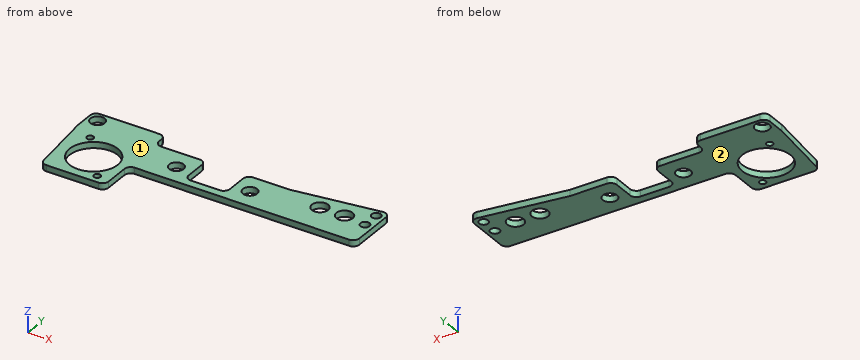
```python
from build123d import *

# Parameters (mm, degrees)
ESQUISSE1_W              = 146
ESQUISSE1_H              = 20
BOSS_EXTRU_1_DEPTH       = 3
ESQUISSE2_R              = 3.5
ENL_V_MAT_EXTRU_3_DEPTH  = 4
ESQUISSE6_W              = 35
ESQUISSE6_H              = 3
BOSS_EXTRU_3_DEPTH       = 8
ESQUISSE8_R              = 3.5
ENL_V_MAT_EXTRU_4_DEPTH  = 8
ESQUISSE7_W              = 35
ESQUISSE7_H              = 3
BOSS_EXTRU_4_DEPTH       = 24
CONG_2_R                 = 3
ESQUISSE10_W             = 20.127249292
ESQUISSE10_H             = 16
ENL_V_MAT_EXTRU_5_DEPTH  = 24
CONG_3_R                 = 3
BOSS_EXTRU_5_DEPTH       = 3
ESQUISSE13_R             = 2.25
ENL_V_MAT_EXTRU_6_DEPTH  = 24
CONG_4_R                 = 3
ESQUISSE16_R             = 11.8
ESQUISSE16_R_2           = 1.6
ENL_V_MAT_EXTRU_7_DEPTH  = 3
ENL_V_MAT_EXTRU_11_DEPTH = 3
CONG_10_R                = 3
ESQUISSE18_R             = 4
ENL_V_MAT_EXTRU_12_DEPTH = 3


with BuildPart() as part:
    # Esquisse1 → Boss.-Extru.1 (new body)
    with BuildSketch(Plane.XY):
        with Locations((73, 10)):
            Rectangle(ESQUISSE1_W, ESQUISSE1_H)
    extrude(amount=BOSS_EXTRU_1_DEPTH)

    # Esquisse2 → Enlèv. mat.-Extru.3 (cut, through all)
    with BuildSketch(Plane.XY.offset(3)):
        with Locations((52, 10)):
            Circle(ESQUISSE2_R)
        with Locations((88, 10)):
            Circle(ESQUISSE2_R)
    extrude(amount=-ENL_V_MAT_EXTRU_3_DEPTH, mode=Mode.SUBTRACT)

    # Esquisse6 → Boss.-Extru.3 (add)
    with BuildSketch(Plane(origin=(0, 20, 0), x_dir=(1, 0, 0), z_dir=(0, 1, 0))):
        with Locations((17.5, -1.5)):
            Rectangle(ESQUISSE6_W, ESQUISSE6_H)
    extrude(amount=BOSS_EXTRU_3_DEPTH)

    # Esquisse8 → Enlèv. mat.-Extru.4 (cut)
    with BuildSketch(Plane.XY.offset(3)):
        with Locations((5, 23)):
            Circle(ESQUISSE8_R)
    extrude(amount=-ENL_V_MAT_EXTRU_4_DEPTH, mode=Mode.SUBTRACT)

    # Esquisse7 → Boss.-Extru.4 (add)
    with BuildSketch(Plane.XZ):
        with Locations((17.5, 1.5)):
            Rectangle(ESQUISSE7_W, ESQUISSE7_H)
    extrude(amount=BOSS_EXTRU_4_DEPTH)

    # Congé2
    cong_2_edges = [part.edges().sort_by_distance(p)[0] for p in [
        (35, 20, 1.5),
        (0, 28, 1.5),
        (35, 28, 1.5),
        (35, -24, 1.5),
        (0, -24, 1.5),
        (35, 0, 1.5),
        (146, 20, 1.5),
        (146, 0, 1.5),
    ]]
    fillet(cong_2_edges, radius=CONG_2_R)

    # Esquisse10 → Enlèv. mat.-Extru.5 (cut)
    with BuildSketch(Plane.XY.offset(3)):
        with Locations((70, 12)):
            Rectangle(ESQUISSE10_W, ESQUISSE10_H)
    extrude(amount=-ENL_V_MAT_EXTRU_5_DEPTH, mode=Mode.SUBTRACT)

    # Congé3
    cong_3_edges = [part.edges().sort_by_distance(p)[0] for p in [
        (80.063624646, 20, 1.5),
        (80.063624646, 4, 1.5),
        (59.936375354, 4, 1.5),
        (59.936375354, 20, 1.5),
    ]]
    fillet(cong_3_edges, radius=CONG_3_R)

    # Esquisse14 → Boss.-Extru.5 (add)
    with BuildSketch(Plane.XY.offset(3)):
        Polygon((146, 10), (146, 26.5), (101, 20), align=None)
    extrude(amount=-BOSS_EXTRU_5_DEPTH)

    # Esquisse13 → Enlèv. mat.-Extru.6 (cut)
    with BuildSketch(Plane.XY.offset(3)):
        with Locations((142, 22)):
            Circle(ESQUISSE13_R)
        with Locations((142, 13.5)):
            Circle(ESQUISSE13_R)
    extrude(amount=-ENL_V_MAT_EXTRU_6_DEPTH, mode=Mode.SUBTRACT)

    # Congé4
    cong_4_edges = [part.edges().sort_by_distance(p)[0] for p in [
        (146, 26.5, 1.5),
    ]]
    fillet(cong_4_edges, radius=CONG_4_R)

    # Esquisse16 → Enlèv. mat.-Extru.7 (cut)
    with BuildSketch(Plane.XY.offset(3)):
        with Locations((19.17587198, -1.870199746)):
            Circle(ESQUISSE16_R)
        with Locations((9.678696735, 10.161451621)):
            Circle(ESQUISSE16_R_2)
        with Locations((28.678696735, -13.838548379)):
            Circle(ESQUISSE16_R_2)
    extrude(amount=-ENL_V_MAT_EXTRU_7_DEPTH, mode=Mode.SUBTRACT)

    # Esquisse17 → Enlèv. mat.-Extru.11 (cut)
    with BuildSketch(Plane.XY.offset(3)):
        Polygon((35, -18), (3.782330551, -18), (0, 15.981074218), (0, -26.941472008), (35, -26.941472008), align=None)
    extrude(amount=-ENL_V_MAT_EXTRU_11_DEPTH, mode=Mode.SUBTRACT)

    # Congé10
    cong_10_edges = [part.edges().sort_by_distance(p)[0] for p in [
        (35, -18, 1.5),
        (0, 15.981074218, 1.5),
        (3.782330551, -18, 1.5),
    ]]
    fillet(cong_10_edges, radius=CONG_10_R)

    # Esquisse18 → Enlèv. mat.-Extru.12 (cut)
    with BuildSketch(Plane.XY.offset(3)):
        with Locations((131, 15)):
            Circle(ESQUISSE18_R)
        with Locations((119, 15)):
            Circle(ESQUISSE18_R)
    extrude(amount=-ENL_V_MAT_EXTRU_12_DEPTH, mode=Mode.SUBTRACT)


solid = part.part
```
Here's how the part is built. I have some questions about the finished solid (model axes, mm). Face numbers are marked on the shaded views. Round coordinates to 2 decimals unless told otherwise and drop trailing zeros. Loops run counter-clockwise (first coordinate to the right, second up) from the corner with the lowest first, then second, coordinate; pieces in that order, holes last. Notation, with made-up numbers: (78.5, 74) -> (127.5, 74) arc R18 cw to (127.5, 79) -> close; hole circle Ø6 at (25, -10). An arc over 180 degrees is marked (long way). Answer as CSV lines item,"result".
1. If we section it at B-B on x = 118: Please give me the cut outline in (y, z), plus the area to 3 significant figures.
Final values:
outline,"(0, 0) -> (11.13, 0) -> (11.13, 3) -> (0, 3) -> close; (18.87, 0) -> (22.46, 0) -> (22.46, 3) -> (18.87, 3) -> close"
area,"44.1 mm^2"
2. If I drill on L1, parallel to X at y = 18, z = 0.35; L2, parallel to X at y = 4.5, z = 1.7; L3, parallel to X at y = 5.5, z = 1.5, over which ranges is the centre line in solid material (lowest first)?
Final values:
L1,"x = 0 to 59.76, 80.24 to 116.35, 121.65 to 128.35, 133.65 to 146"
L2,"x = 1.28 to 9.24, 29.11 to 61.28, 78.72 to 146"
L3,"x = 1.17 to 9.96, 28.39 to 60.34, 79.66 to 146"
3. For pin 1 (0.6 mm diameter, centred on y = 24.5, z = 1, fed in from +X); pin 2 (1.5 mm diameter, centred on y = -11, z = 1.5, fed in from +X); pin 3 (0.9 mm diameter, centred on x = 76, z = 1, fed in from -Y), each with a flat end and sliding along its axis, tell me the tip position at first contact or that it passes through.
Final values:
pin 1,"stops at x = 145.76"
pin 2,"stops at x = 35"
pin 3,"stops at y = 0"
4. Thinking about a two-plate mould opening in Z: for the marked faces 1 and 2, which applies, released by +Z, released by -Z, zero draft, split by the parting line, or undercut?
Final values:
face 1,"released by +Z"
face 2,"released by -Z"
5. If we section it at C-C on z = 2.5: Count the separate pieces of the cut face and the enclosed holes in it, plus the area to 3 significant figures.
Final values:
separate pieces,"1"
enclosed holes,"10"
area,"2,880 mm^2"
6. If we section it at A-A on x = 88: Please give me the cut outline in (y, z), plus the area to 3 significant figures.
Final values:
outline,"(0, 0) -> (6.5, 0) -> (6.5, 3) -> (0, 3) -> close; (13.5, 0) -> (20, 0) -> (20, 3) -> (13.5, 3) -> close"
area,"39.0 mm^2"
